Work out the finished part from the listing and answer in its coordinate system (mm). A direction names the side the tool comes from. Round coordinates to 2 decimals unless told otherwise and drop trailing zeros. Loops run counter-clockwise (first coordinate to the right, second up) from the corner with the lowest first, then second, coordinate; pieces in that order, holes last.
```python
from build123d import *

# Parameters (mm, degrees)
SKETCH1_W           = 508
SKETCH1_H           = 393.7
SKETCH1_W_2         = 479.425
SKETCH1_H_2         = 365.125
BOSS_EXTRUDE1_DEPTH = 54.356
SKETCH2_W           = 393.7
SKETCH2_H           = 12.7
BOSS_EXTRUDE2_DEPTH = 508
FILLET1_R           = 6.35
FILLET2_R           = 6.35


with BuildPart() as part:
    # Sketch1 → Boss-Extrude1 (new body)
    with BuildSketch(Plane(origin=(0, 0, 0), x_dir=(1, 0, 0), z_dir=(0, 1, 0))):
        with Locations((254, 196.85)):
            Rectangle(SKETCH1_W, SKETCH1_H)
        with Locations((254, 196.8373)):
            Rectangle(SKETCH1_W_2, SKETCH1_H_2, mode=Mode.SUBTRACT)
    extrude(amount=BOSS_EXTRUDE1_DEPTH)

    # Sketch2 → Boss-Extrude2 (add)
    with BuildSketch(Plane(origin=(508, 0, 0), x_dir=(0, 0, -1), z_dir=(1, 0, 0))):
        with Locations((196.85, 48.006)):
            Rectangle(SKETCH2_W, SKETCH2_H)
    extrude(amount=-BOSS_EXTRUDE2_DEPTH)

    # Fillet1
    fillet1_edges = [part.edges().sort_by_distance(p)[0] for p in [
        (508, 54.356, -196.85),
        (254, 54.356, -393.7),
        (0, 54.356, -196.85),
        (254, 54.356, 0),
        (0, 27.178, -393.7),
        (508, 27.178, -393.7),
        (508, 27.178, 0),
        (0, 27.178, 0),
    ]]
    fillet(fillet1_edges, radius=FILLET1_R)

    # Fillet2
    fillet2_edges = [part.edges().sort_by_distance(p)[0] for p in [
        (493.7125, 20.828, -379.3998),
        (14.2875, 20.828, -379.3998),
        (254, 41.656, -379.3998),
        (493.7125, 20.828, -14.2748),
        (14.2875, 20.828, -14.2748),
        (254, 41.656, -14.2748),
        (14.2875, 41.656, -196.8373),
        (493.7125, 41.656, -196.8373),
    ]]
    fillet(fillet2_edges, radius=FILLET2_R)


solid = part.part
```
1. Find section C-C (x = 352). Write down the section's boundary in (y, z), then the cut area to 3 significant figures.
Answer key:
outline: (0, -393.7) - (48.01, -393.7) arc R6.35 ccw to (54.36, -387.35) - (54.36, -6.35) arc R6.35 ccw to (48.01, 0) - (0, 0) - (0, -14.27) - (35.31, -14.27) arc R6.35 cw to (41.66, -20.62) - (41.66, -373.05) arc R6.35 cw to (35.31, -379.4) - (0, -379.4) - close
area: 6,190 mm2
2. Find section A-A (z = -186). Write down the section's boundary in (x, y), then the cut area to 3 significant figures.
Answer key:
outline: (0, 0) - (14.29, 0) - (14.29, 35.31) arc R6.35 cw to (20.64, 41.66) - (487.36, 41.66) arc R6.35 cw to (493.71, 35.31) - (493.71, 0) - (508, 0) - (508, 48.01) arc R6.35 ccw to (501.65, 54.36) - (6.35, 54.36) arc R6.35 ccw to (0, 48.01) - close
area: 7,640 mm2
3. Which of the six approach directions +Z, -Z, +X, -X, +Y, -Y give full straight-line access (tool end or side, diameter ignored) to faces 1 (the face through (234, 0, -8)), 2 (the face through (251, 17, -14.275))?
Answer key:
face 1: +Z, -Z, +X, -X, -Y
face 2: -Y
4. Determine the mould class of faces 3 (the face through (251, 54.356, -200)), 4 (the face through (508, 24, -194)), 5 (the face through (14.287, 17, -194)) for opening direction X: +X half, -X half, draft (parallel to the pull), parting line (faces both ways), or undercut.
Answer key:
face 3: draft
face 4: +X half
face 5: undercut
5. Find section B-B (y = 9). Write down the section's boundary in (x, z).
Answer key:
outline: (0, -387.35) arc R6.35 ccw to (6.35, -393.7) - (501.65, -393.7) arc R6.35 ccw to (508, -387.35) - (508, -6.35) arc R6.35 ccw to (501.65, 0) - (6.35, 0) arc R6.35 ccw to (0, -6.35) - close; hole (14.29, -373.05) arc R6.35 ccw to (20.64, -379.4) - (487.36, -379.4) arc R6.35 ccw to (493.71, -373.05) - (493.71, -20.62) arc R6.35 ccw to (487.36, -14.27) - (20.64, -14.27) arc R6.35 ccw to (14.29, -20.62) - close
6. Consider probe 1 along Z at (x, y) = (46, 10); probe 2 along X at (y, z) = (35, -224.5); probe 3 along X at (y, z) = (41, -70.5). Determine where each line is inside the solid, lowest interval first.
Answer key:
probe 1: z = -393.7 to -379.4, -14.27 to 0
probe 2: x = 0 to 14.29, 493.71 to 508
probe 3: x = 0 to 17.83, 490.17 to 508
